Geometry check sheet. Reference: drawing and pictorial views, mm from the part's lowest x, y, z. Give positions to 0.01 mm unless a question says otherwise; leave off trailing zeros. Order: outer loops, then holes, each group sorted by start corner. A loop starts at its lowest first (then second) coordinate and runs counter-clockwise, first axis right, second up. Notation, with made-up numbers: M 62,49 L 116,49 A31 ccw 116,79 Z; hole C -27,80.25 d9. An arc over 180 degrees is marked long. Answer as CSV lines item,"result". Start each with the question number.
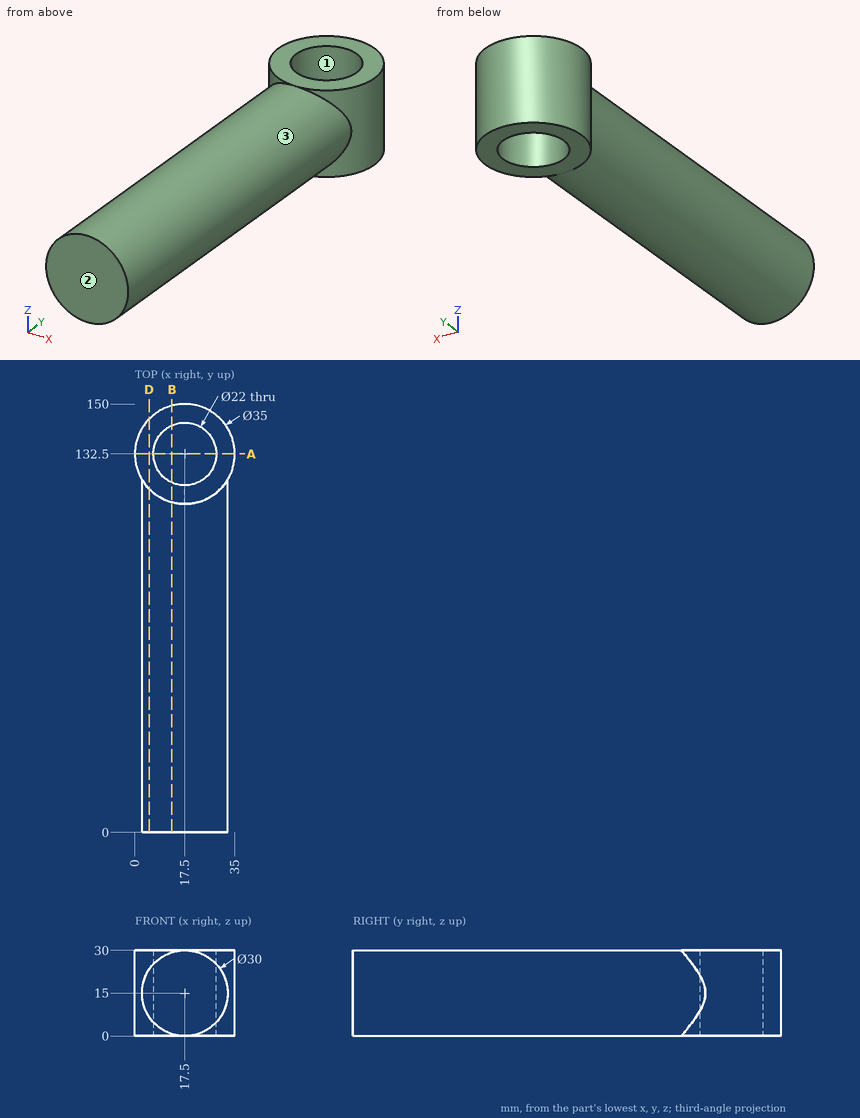
Item 1: Draft check along X on the marked faces 1, 2 and 3. Enter one of: pulls with the +X half, pulls with the -X half, needs draft (parallel to the pull), parting line crosses it, or undercut.
Item 2: Scan lines: line 1 along X through (y, z) = (132, 12); line 2 along Z through (x, y) = (18, 89); line 3 along X through (y, z) = (141, 25). Record each from-to range of solid material in increasing order.
Item 3: Section check D-D on x = 5. Record the boundary of the cut face in (y, z).
Item 4: Section check B-B on x = 13. Record the boundary of the cut face in (y, z), then the cut area to 3 significant figures.
Item 5: Section check A-A on y = 132.5. Record the boundary of the cut face in (x, z), then the cut area to 3 significant figures.
Item 6: Depth check by flat-ended pin: pin 1 Ø1.5 at (x, y) = (27, 31) entering from +Z; pin 2 Ø1 at (x, z) = (16.5, 10) entering from +Y; pin 3 Ø5 at (x, z) = (5, 25.5) entering from +Y. Enter the tip coordinate at first touch or a pass-through.
Numbers:
1,face 1,"undercut"
1,face 2,"needs draft"
1,face 3,"parting line crosses it"
2,line 1,"0.01 to 6.51, 28.49 to 34.99"
2,line 2,"0.01 to 29.99"
2,line 3,"2.2 to 10.52, 24.48 to 32.8"
3,outline,"M 0,6.71 L 120.25,6.71 L 120.25,0 L 144.75,0 L 144.75,30 L 120.25,30 L 120.25,23.29 L 0,23.29 Z"
4,outline,"M 0,0.69 L 115.59,0.69 L 115.59,0 L 122.46,0 L 122.46,30 L 115.59,30 L 115.59,29.31 L 0,29.31 Z; M 142.54,0 L 149.41,0 L 149.41,30 L 142.54,30 Z"
4,area,"3,720 mm2"
5,outline,"M 0,0 L 6.5,0 L 6.5,30 L 0,30 Z; M 28.5,0 L 35,0 L 35,30 L 28.5,30 Z"
5,area,"390 mm2"
6,pin 1,"z = 27.18"
6,pin 2,"y = 149.99"
6,pin 3,"y = 146.86"
